Input: part model. Units: mm. Frame: model coordinates. A direction names the side the tool comes from. Coordinates: 2 decimals unless noted, no trailing zeros. Loops run counter-clockwise (first coordinate to the right, second up) from the corner with the lowest first, then second, coordinate; pieces in that order, holes last.
```python
from build123d import *

# Parameters (mm, degrees)
SKETCH1_W           = 30
SKETCH1_H           = 6
BOSS_EXTRUDE1_DEPTH = 6
SKETCH2_R           = 1.45
CUT_EXTRUDE1_DEPTH  = 32.176914536
SKETCH3_W           = 2.6
SKETCH3_H           = 5.5
CUT_EXTRUDE2_DEPTH  = 32.176914536
SKETCH4_W           = 7
SKETCH4_H           = 2
BOSS_EXTRUDE2_DEPTH = 6
FILLET1_R           = 2
FILLET2_R           = 2


with BuildPart() as part:
    # Sketch1 → Boss-Extrude1 (new body)
    with BuildSketch(Plane.XY):
        with Locations((15, -3)):
            Rectangle(SKETCH1_W, SKETCH1_H)
    extrude(amount=BOSS_EXTRUDE1_DEPTH)

    # Sketch2 → Cut-Extrude1 (cut, through all)
    with BuildSketch(Plane(origin=(30, 0, 0), x_dir=(0, 0, -1), z_dir=(1, 0, 0))):
        with Locations((-3, -3)):
            Circle(SKETCH2_R)
    extrude(amount=-CUT_EXTRUDE1_DEPTH, mode=Mode.SUBTRACT)

    # Sketch3 → Cut-Extrude2 (cut, through all)
    with BuildSketch(Plane(origin=(0, 0, 0), x_dir=(1, 0, 0), z_dir=(0, 1, 0))):
        with Locations((7.3, -3)):
            Rectangle(SKETCH3_W, SKETCH3_H)
        with Locations((22.7, -3)):
            Rectangle(SKETCH3_W, SKETCH3_H)
    extrude(amount=-CUT_EXTRUDE2_DEPTH, mode=Mode.SUBTRACT)

    # Sketch4 → Boss-Extrude2 (add)
    with BuildSketch(Plane(origin=(0, 0, 0), x_dir=(1, 0, 0), z_dir=(0, 1, 0))):
        with Locations((7.5, -7)):
            Rectangle(SKETCH4_W, SKETCH4_H)
        with Locations((22.5, -7)):
            Rectangle(SKETCH4_W, SKETCH4_H)
        with Locations((7.5, 1)):
            Rectangle(SKETCH4_W, SKETCH4_H)
        with Locations((22.5, 1)):
            Rectangle(SKETCH4_W, SKETCH4_H)
    extrude(amount=-BOSS_EXTRUDE2_DEPTH)

    # Fillet1
    fillet1_edges = [part.edges().sort_by_distance(p)[0] for p in [
        (26, -3, -2),
        (4, -3, -2),
        (11, -3, -2),
        (19, -3, -2),
        (26, -3, 8),
        (19, -3, 8),
        (11, -3, 8),
        (4, -3, 8),
    ]]
    fillet(fillet1_edges, radius=FILLET1_R - 0.0001)  # a hair under: the kernel refuses the full size

    # Fillet2
    fillet2_edges = [part.edges().sort_by_distance(p)[0] for p in [
        (4, -3, 6),
        (11, -3, 6),
        (19, -3, 6),
        (26, -3, 6),
        (4, -3, 0),
        (11, -3, 0),
        (19, -3, 0),
        (26, -3, 0),
    ]]
    fillet(fillet2_edges, radius=FILLET2_R)


solid = part.part
```
Item 1: Section query B-B (x = 13.5). Output: boundary loops of the cut face in (y, z), then the cut area to 3 significant figures.
Result:
outline: (-6, 0) - (0, 0) - (0, 6) - (-6, 6) - close; hole circle Ø2.9 at (-3, 3)
area: 29.4 mm2
Item 2: Mould query, pull axis Y, two halves, no side actions, for faces 1 (the face through (3.04, -2.02, 4.07)), 2 (the face through (19.987, -3.042, 7.725)), 3 (the face through (15, 0, 3)). Classes: +Y half, -Y half, draft (parallel to the pull), parting line (faces both ways), or undercut.
Result:
face 1: undercut
face 2: draft
face 3: +Y half
Item 3: Reachability of faces 4 (the face through (29, -3, 0)), 5 (the face through (7, -3, 0.25)), 6 (the face through (10.013, -3.042, -1.725)), 7 (the face through (24.99, -3.04, 7.74)) from +Z, -Z, +X, -X, +Y, -Y: full face, straight path, thin tool, end or side. Return the list, or none.
Result:
face 4: -Z, +X, +Y, -Y
face 5: +Y, -Y
face 6: -Z, +Y, -Y
face 7: +Z, +X, +Y, -Y
Item 4: Line query: L1, parallel to X at y = -1, z = 1.75; L2, parallel to Y at x = 16, z = 3; L3, parallel to Z at x = 21.5, y = -2.25. Output: solid intervals per line, ascending.
Result:
L1: x = 0 to 6, 8.6 to 21.4, 24 to 30
L2: y = -6 to -4.45, -1.55 to 0
L3: z = -2 to 0.25, 5.75 to 8
Item 5: Section query D-D (y = -0.5). Count the separate pieces of the cut face and the enclosed holes in it, then the cut area to 3 significant figures.
Result:
separate pieces: 1
enclosed holes: 2
area: 203 mm2
Item 6: Section query C-C (z = 0.75). Output: boundary loops of the cut face in (x, y), then the cut area to 3 significant figures.
Result:
outline: (0, -6) - (6, -6) - (6, 0) - (0, 0) - close; (8.6, -6) - (21.4, -6) - (21.4, 0) - (8.6, 0) - close; (24, -6) - (30, -6) - (30, 0) - (24, 0) - close
area: 149 mm2
Item 7: Contact query for flat-ended pins moving along their axis: P1, Ø1, axis at x = 4.5, y = -4, coming from the -Z side; P2, Ø0.8, axis at x = 29.5, y = -1.5, coming from the -Z side; P3, Ø2, axis at x = 2, y = -3.5, coming from the -Z side; P4, Ø2.5, axis at y = -3, z = 3, coming from the +X side. Output: stop coordinate, or through.
Result:
P1: stops at z = -1.73
P2: stops at z = 0
P3: stops at z = -0.05
P4: passes through
Item 8: Section query A-A (z = 3). Output: boundary loops of the cut face in (x, y).
Result:
outline: (0, -6) - (6, -6) - (6, -4.45) - (0, -4.45) - close; (0, -1.55) - (6, -1.55) - (6, 0) - (0, 0) - close; (8.6, -6) - (21.4, -6) - (21.4, -4.45) - (8.6, -4.45) - close; (8.6, -1.55) - (21.4, -1.55) - (21.4, 0) - (8.6, 0) - close; (24, -6) - (30, -6) - (30, -4.45) - (24, -4.45) - close; (24, -1.55) - (30, -1.55) - (30, 0) - (24, 0) - close
